Source: CAD feature listing. Evaluate the final solid. Frame: model axes, mm. Face numbers are marked on the shaded views. A direction names the side the tool comes from. Give positions to 0.01 mm unless a question says otherwise; leave off trailing zeros. Loops run counter-clockwise (first coordinate to the right, second up) from the corner with the lowest first, then second, coordinate; pieces in that order, holes last. Notation, with made-up numbers: (68.5, 84.25) -> (102.5, 84.25) arc R19 ccw to (102.5, 119.25) -> close; hole circle Ø4 at (46.25, 78). An arc over 180 degrees is marked (long way). Put each result on its own line as item: value.
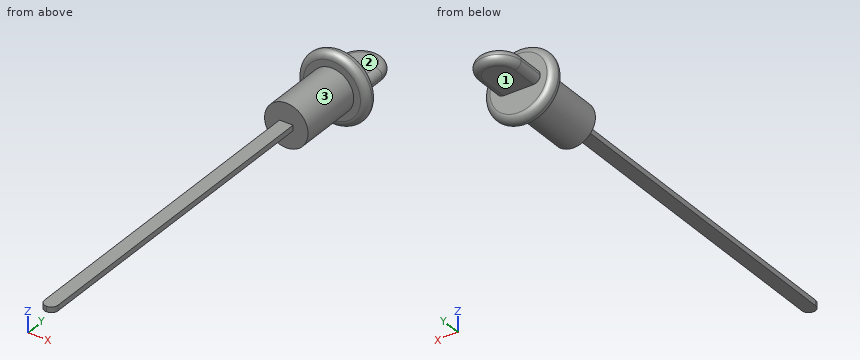
```python
from build123d import *

# Parameters (mm, degrees)
SKETCH1_R           = 5.08
BOSS_EXTRUDE1_DEPTH = 15.24
SKETCH2_R           = 8.255
BOSS_EXTRUDE2_DEPTH = 3.175
BOSS_EXTRUDE3_DEPTH = 1.5875
FILLET1_R           = 1.5875
SKETCH4_W           = 3.175
SKETCH4_H           = 1.27
BOSS_EXTRUDE4_DEPTH = 80.01
FILLET3_R           = 1.5875


with BuildPart() as part:
    # Sketch1 → Boss-Extrude1 (new body)
    with BuildSketch(Plane(origin=(0, 0, 0), x_dir=(1, 0, 0), z_dir=(0, 1, 0))):
        with Locations(Location((0, 0, 0), (0, 0, 270))):
            Circle(SKETCH1_R)
    extrude(amount=-BOSS_EXTRUDE1_DEPTH)

    # Sketch2 → Boss-Extrude2 (add)
    with BuildSketch(Plane(origin=(0, 0, 0), x_dir=(1, 0, 0), z_dir=(0, 1, 0))):
        with Locations(Location((0, 0, 0), (0, 0, 270))):
            Circle(SKETCH2_R)
    extrude(amount=BOSS_EXTRUDE2_DEPTH)

    # Sketch3 → Boss-Extrude3 (add, symmetric)
    with BuildSketch(Plane.XY):
        with BuildLine():
            Line((5.08, 3.175), (-5.08, 3.175))
            Line((-5.08, 3.175), (-5.08, 9.525))
            ThreePointArc((-5.08, 9.525), (0, 14.605), (5.08, 9.525))
            Line((5.08, 9.525), (5.08, 3.175))
        make_face()
    extrude(amount=BOSS_EXTRUDE3_DEPTH, both=True)

    # Fillet1
    fillet1_edges = [part.edges().sort_by_distance(p)[0] for p in [
        (5.08, 6.35, -1.5875),
        (-5.08, 6.35, -1.5875),
        (-5.08, 6.35, 1.5875),
        (0, 14.605, 1.5875),
        (0, 0, -8.255),
        (0, 3.175, -8.255),
        (0, 14.605, -1.5875),
        (5.08, 6.35, 1.5875),
    ]]
    fillet(fillet1_edges, radius=FILLET1_R - 0.0001)  # a hair under: the kernel refuses the full size

    # Sketch4 → Boss-Extrude4 (add)
    with BuildSketch(Plane.XZ.offset(15.24)):
        Rectangle(SKETCH4_W, SKETCH4_H)
    extrude(amount=BOSS_EXTRUDE4_DEPTH)

    # Fillet3
    fillet3_edges = [part.edges().sort_by_distance(p)[0] for p in [
        (-1.5875, -95.25, 0),
        (1.5875, -95.25, 0),
    ]]
    fillet(fillet3_edges, radius=FILLET3_R - 0.0001)  # a hair under: the kernel refuses the full size


solid = part.part
```
(1) Section A-A on y = -36. Return loops of the section in (x, z) (1 decimal).
Calculated:
outline: (-1.6, -0.6) -> (1.6, -0.6) -> (1.6, 0.6) -> (-1.6, 0.6) -> close
(2) Reachability of the marked faces 1, 2 and 3 from +Z, -Z, +X, -X, +Y, -Y: full face, straight path, thin tool, end or side. Return the list, or none.
Calculated:
face 1: -Z, +X, -X, +Y
face 2: +Z, +X, -X, +Y
face 3: -Y
(3) Line query: probe 1 along Z at (x, y) = (1, 9.5); probe 2 along Y at (x, z) = (-5.5, -1) (3 decimals). Output: solid intervals per line, ascending. Write a range as from..to.
Calculated:
probe 1: z = -1.59..1.59
probe 2: y = 0..3.175
(4) First-contact query: P1, Ø8, axis at y = -73, z = -5, coming from the -X side; P2, Ø1.6, axis at x = 0.5, y = -42, coming from the -Z side (3 decimals); P3, Ø2, axis at x = 1, y = 9, coming from the +Z side; P4, Ø2, axis at x = -1, z = 0, coming from the -Y side. Flat tips, straight axial feed; report the tip coordinate or a pass-through.
Calculated:
P1: passes through
P2: stops at z = -0.635
P3: stops at z = 1.59
P4: stops at y = -95.25
